Model file for the job. Use its own axes, mm. A direction names the side the tool comes from. Give positions to 0.01 mm unless a question says otherwise; leave off trailing zeros. Loops run counter-clockwise (first coordinate to the right, second up) from the corner with the lowest first, then second, coordinate; pieces in that order, holes last. Notation, with made-up numbers: (53, 68) -> (62, 68) arc R29 ccw to (62, 100) -> close; hole circle Ø11 at (84, -29.75). An arc over 180 degrees is marked (long way). Use CSV: the item, a comma, the result in double quotes. Start each with the question number.
(1) Flat gauge pins, fed straight in: pin 1 (0.9 mm diameter, centred on x = 27, z = 1, fed in from +Y); pin 2 (10 mm diameter, centred on x = 20.5, y = -21, fed in from -Z); pin 3 (0.9 mm diameter, centred on y = 1.5, z = 2, fed in from +X) (3 decimals). Where does each tip first touch, or does it go through?
(2) Cut at C-C on z = 0.45. Write the cut outline in (x, y) (3 decimals).
(3) 3-axis set-ups, long thin cutter, end or side, ignore diameter. For faces 1 (the flat face through (29, 0, 1)), 2 (the flat face through (2, -40, 1)), 3 (the flat face through (12.435, 2, 1)): which of +Z, -Z, +X, -X, +Y, -Y reach the whole face in a straight line?
(4) Cut at A-A on x = 32. Write the cut outline in (y, z), then the cut area to 3 significant figures.
(5) Cut at B-B on y = -54. Write the cut outline in (x, z).
(6) Cut at D-D on x = 24. Write the cut outline in (y, z), then the cut area to 3 significant figures.
(7) Drill centre lines: probe 1 along X at (y, z) = (-33, 1.9); probe 2 along Y at (x, z) = (32, 1.35); probe 3 along Y at (x, z) = (23, 2.85). Where is each one in solid material? Low to high.
(8) Pull direction X, two halves, no side cores. Call faces 4 (the flat face through (34.87, -41, 1)), 5 (the flat face through (6, 0, 1)), 6 (the flat face through (32.87, -40, 1)): pulls with the +X half, pulls with the -X half, needs draft (parallel to the pull), parting line crosses it, or undercut.
from build123d import *

# Parameters (mm, degrees)
EXTRUDE_1_DEPTH = 3


with BuildPart() as part:
    # 草图1 → 凸台-拉伸1 (new body)
    with BuildSketch(Plane.XY):
        Polygon((0, 0), (0, -40), (2, -40), (2, -25), (5, -25), (5, -40), (17.435, -40), (17.435, 0), (12.435, 0), align=None)
        Polygon((2, -40), (0, -40), (0, -80), (17.435, -80), (17.435, -40), (5, -40), (5, -55), (2, -55), align=None)
        Polygon((17.435, -40), (17.435, -80), (34.87, -80), (34.87, -40), (32.87, -40), (32.87, -55), (29.87, -55), (29.87, -40), align=None)
        Polygon((17.435, 0), (17.435, -40), (29.87, -40), (29.87, -25), (32.87, -25), (32.87, -40), (34.87, -40), (34.87, 0), (22.435, 0), align=None)
        Polygon((12.435, 3), (12.435, 0), (17.435, 0), (22.435, 0), (22.435, 3), align=None)
    extrude(amount=EXTRUDE_1_DEPTH)


solid = part.part
Check result:
1,pin 1,"y = 0"
1,pin 2,"z = 0"
1,pin 3,"x = 22.435"
2,outline,"(0, -80) -> (34.87, -80) -> (34.87, 0) -> (22.435, 0) -> (22.435, 3) -> (12.435, 3) -> (12.435, 0) -> (0, 0) -> close; hole (2, -55) -> (5, -55) -> (5, -25) -> (2, -25) -> close; hole (29.87, -55) -> (32.87, -55) -> (32.87, -25) -> (29.87, -25) -> close"
3,face 1,"+Z, -Z, +X, +Y"
3,face 2,"+Z, -Z"
3,face 3,"+Z, -Z, -X, +Y"
4,outline,"(-80, 0) -> (-55, 0) -> (-55, 3) -> (-80, 3) -> close; (-25, 0) -> (0, 0) -> (0, 3) -> (-25, 3) -> close"
4,area,"150 mm²"
5,outline,"(0, 0) -> (2, 0) -> (2, 3) -> (0, 3) -> close; (5, 0) -> (29.87, 0) -> (29.87, 3) -> (5, 3) -> close; (32.87, 0) -> (34.87, 0) -> (34.87, 3) -> (32.87, 3) -> close"
6,outline,"(-80, 0) -> (0, 0) -> (0, 3) -> (-80, 3) -> close"
6,area,"240 mm²"
7,probe 1,"0 to 2, 5 to 29.87, 32.87 to 34.87"
7,probe 2,"-80 to -55, -25 to 0"
7,probe 3,"-80 to 0"
8,face 4,"pulls with the +X half"
8,face 5,"needs draft"
8,face 6,"undercut"
